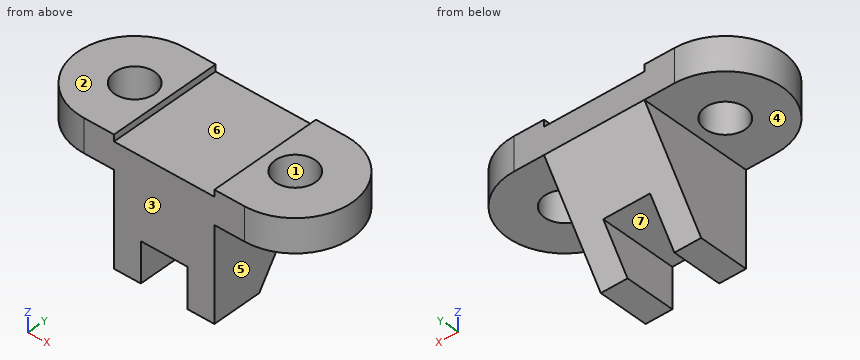
from build123d import *

# Parameters (mm, degrees)
EXTRUDE_1_DEPTH          = 10
SKETCH_2_R               = 6
CUT_EXTRUDE_1_DEPTH      = 18
SKETCH_3_W               = 30
SKETCH_3_H               = 34
EXTRUDE_2_DEPTH          = 28
CUT_EXTRUDE_2_DEPTH      = 14
CUT_EXTRUDE_2_DEPTH_BACK = 45
SKETCH_4_W               = 14
SKETCH_4_H               = 24
CUT_EXTRUDE_3_DEPTH      = 45
SKETCH_6_W               = 30
SKETCH_6_H               = 4
CUT_EXTRUDE_5_DEPTH      = 34


with BuildPart() as part:
    # 草图1 → 凸台-拉伸1 (new body)
    with BuildSketch(Plane.XY):
        with BuildLine():
            Line((24, -17), (-24, -17))
            ThreePointArc((-24, -17), (-41, 0), (-24, 17))
            Line((-24, 17), (24, 17))
            ThreePointArc((24, 17), (41, 0), (24, -17))
        make_face()
    extrude(amount=EXTRUDE_1_DEPTH)

    # 草图2 → 切除-拉伸1 (cut)
    with BuildSketch(Plane.XY):
        with Locations((-24, 0)):
            Circle(SKETCH_2_R)
        with Locations((24, 0)):
            Circle(SKETCH_2_R)
    extrude(amount=CUT_EXTRUDE_1_DEPTH, mode=Mode.SUBTRACT)

    # 草图3 → 凸台-拉伸2 (add)
    with BuildSketch(Plane.XY):
        Rectangle(SKETCH_3_W, SKETCH_3_H)
    extrude(amount=-EXTRUDE_2_DEPTH)

    # 草图4 → 切除-拉伸2 (cut, two sides: drawn at the far end of the back side and taken through both)
    with BuildSketch(Plane.XZ.offset(17).offset(-CUT_EXTRUDE_2_DEPTH_BACK)):
        with Locations((0, -28)):
            Rectangle(SKETCH_4_W, SKETCH_4_H)
    extrude(amount=CUT_EXTRUDE_2_DEPTH + CUT_EXTRUDE_2_DEPTH_BACK, mode=Mode.SUBTRACT)

    # 草图5 → 切除-拉伸3 (cut)
    with BuildSketch(Plane.ZY.offset(15)):
        Polygon((0, 17), (-28, 17), (-28, -2), align=None)
    extrude(amount=-CUT_EXTRUDE_3_DEPTH, mode=Mode.SUBTRACT)

    # 草图6 → 切除-拉伸5 (cut)
    with BuildSketch(Plane(origin=(0, 17, 0), x_dir=(1, 0, 0), z_dir=(0, 1, 0))):
        with Locations((0, -10)):
            Rectangle(SKETCH_6_W, SKETCH_6_H)
    extrude(amount=-CUT_EXTRUDE_5_DEPTH, mode=Mode.SUBTRACT)


solid = part.part
Read the model definition and answer for the solid it produces. Units are mm, in the model's axes. Face numbers are marked on the shaded views. A direction names the side the tool comes from. Round coordinates to 2 decimals unless told otherwise and drop trailing zeros. Order: outer loops, then holes, each group sorted by start corner. A loop starts at its lowest first (then second) coordinate and runs counter-clockwise, first axis right, second up.
1) The part is cut by section A-A on z = -17.5. Write down the section's boundary in (x, y) (3 decimals).
2) The part is cut by section C-C on y = -1. Write down the section's boundary in (x, z), plus the area to 3 significant figures.
3) The part is cut by section B-B on y = -8. Write down the section's boundary in (x, z).
4) For the marked faces 4, 5, 6 and 7, determine the directions among +Z, -Z, +X, -X, +Y, -Y from which every point of the face is accessible in a straight line to the end or side of a thin tool.
5) Flat-ended cylindrical pins translate along their axes: pin 1 (0.6 mm diameter, centred on y = 7.5, z = 9.5, fed in from -X); pin 2 (2 mm diameter, centred on y = 6.5, z = 9, fed in from +X); pin 3 (4 mm diameter, centred on x = -10, z = -9.5, fed in from +Y); pin 4 (15.5 mm diameter, centred on x = -2.5, y = -4, fed in from -Z). Find the tip coordinate at first contact, or state that the pin passes through.
6) The mould has two halves that part along Y. Classify the marked faces 1, 2 and 3: released by +Y, released by -Y, zero draft, split by the parting line, or undercut.
7) Straight lines are drawn through the part: L1, parallel to X at y = 0, z = 5.5; L2, parallel to X at y = -6, z = -22.5; L3, parallel to Y at x = -24, z = 6. For each, find the intervals that lie inside material, in ascending order.
8) The part is cut by section D-D on z = -10.5. Write down the section's boundary in (x, y) (3 decimals).
Resolved:
1. outline: (-15, -17) - (-7, -17) - (-7, 5.125) - (-15, 5.125) - close; (7, -17) - (15, -17) - (15, 5.125) - (7, 5.125) - close
2. outline: (-40.97, 0) - (-29.92, 0) - (-29.92, 10) - (-40.97, 10) - close; (-18.08, 0) - (-15, 0) - (-15, -26.53) - (-7, -26.53) - (-7, -16) - (7, -16) - (7, -26.53) - (15, -26.53) - (15, 0) - (18.08, 0) - (18.08, 10) - (15, 10) - (15, 8) - (-15, 8) - (-15, 10) - (-18.08, 10) - close; (29.92, 0) - (40.97, 0) - (40.97, 10) - (29.92, 10) - close
2. area: 1,170 mm2
3. outline: (-39, 0) - (-15, 0) - (-15, -28) - (-7, -28) - (-7, -16) - (7, -16) - (7, -28) - (15, -28) - (15, 0) - (39, 0) - (39, 10) - (15, 10) - (15, 8) - (-15, 8) - (-15, 10) - (-39, 10) - close
4. face 4: -Z, -X, +Y, -Y
4. face 5: -Z, +X, +Y, -Y
4. face 6: +Z, +Y, -Y
4. face 7: -Z, +Y, -Y
5. pin 1: stops at x = -39.4
5. pin 2: stops at x = 40.09
5. pin 3: stops at y = 11.91
5. pin 4: stops at z = -28
6. face 1: undercut
6. face 2: zero draft
6. face 3: released by -Y
7. L1: x = -41 to -30, -18 to 18, 30 to 41
7. L2: x = -15 to -7, 7 to 15
7. L3: y = -17 to -6, 6 to 17
8. outline: (-15, -17) - (15, -17) - (15, 9.875) - (-15, 9.875) - close
